```python
from build123d import *

# Parameters (mm, degrees)
ESBO_O1_W                  = 148
ESBO_O1_H                  = 130
RESSALTO_EXTRUS_O1_DEPTH   = 10
FURO_COM_FOLGA_DE_M3X0_5_D = 3.4
ESBO_O5_R                  = 5
CORTE_EXTRUS_O1_DEPTH      = 4.5
CORTE_EXTRUS_O2_REACH      = 205.463
ESBO_O6_R                  = 4


with BuildPart() as part:
    # Esboço1 → Ressalto-extrusão1 (new body)
    with BuildSketch(Plane.XY):
        with Locations((-0.0034, 124.2634)):
            Rectangle(ESBO_O1_W, ESBO_O1_H)
    extrude(amount=RESSALTO_EXTRUS_O1_DEPTH)

    # Furo com folga de M3X0.5 (through all)
    with Locations(Plane.XY.offset(10)):
        with Locations((38.5, 67), (-38.5068, 67), (65.5, 124), (-65.5068, 124), (-38.5068, 181), (38.5, 181)):
            Hole(FURO_COM_FOLGA_DE_M3X0_5_D / 2)

    # Esboço5 → Corte-extrusão1 (cut)
    with BuildSketch(Plane.XY.offset(10)):
        with Locations((-18.7634, 111.5234)):
            Circle(ESBO_O5_R)
        with Locations((18.8366, 137.5034)):
            Circle(ESBO_O5_R)
    extrude(amount=-CORTE_EXTRUS_O1_DEPTH, mode=Mode.SUBTRACT)

    # Esboço6 → Corte-extrusão2 (cut, up to next)
    with BuildSketch(Plane.XY.offset(10), mode=Mode.PRIVATE) as corte_extrus_o2_sk1:
        with Locations((-18.7634, 111.5234)):
            Circle(ESBO_O6_R)
    corte_extrus_o2_tool1 = extrude(corte_extrus_o2_sk1.sketch, amount=-CORTE_EXTRUS_O2_REACH, mode=Mode.PRIVATE) & part.part
    # Esboço6 → Corte-extrusão2 (cut, up to next)
    with BuildSketch(Plane.XY.offset(10), mode=Mode.PRIVATE) as corte_extrus_o2_sk2:
        with Locations((18.8366, 137.5034)):
            Circle(ESBO_O6_R)
    corte_extrus_o2_tool2 = extrude(corte_extrus_o2_sk2.sketch, amount=-CORTE_EXTRUS_O2_REACH, mode=Mode.PRIVATE) & part.part
    add(corte_extrus_o2_tool1.solids().sort_by_distance((-18.7634, 111.5234, 10))[0], mode=Mode.SUBTRACT)
    add(corte_extrus_o2_tool2.solids().sort_by_distance((18.8366, 137.5034, 10))[0], mode=Mode.SUBTRACT)


solid = part.part
```
Check sheet for the modelled part. Datum: model origin and axes. Units: mm. A direction names the side the tool comes from. Round coordinates to 2 decimals unless told otherwise and drop trailing zeros. Loops run counter-clockwise (first coordinate to the right, second up) from the corner with the lowest first, then second, coordinate; pieces in that order, holes last. Notation, with made-up numbers: (39.5, 28.25) -> (74.5, 28.25) arc R16 ccw to (74.5, 36.25) -> close; hole circle Ø4 at (18, -8.75). An arc over 180 degrees is marked (long way). Write item = value, one per line. Start each with the question number.
1) Release check for a two-part mould opening along Y. For faces 3 (the cylindrical face through (-19.28, 115.49, 2.79)), 4 (the flat face through (73.997, 123, 5)), 5 (the flat face through (-1, 189.263, 5)), 6 (the cylindrical face through (-63.81, 124.07, 4.93)) record: released by +Y, released by -Y, zero draft, split by the parting line, or undercut.
2) Sectioned sample at B-B, the plane y = 124. Record the cut outline in (x, z).
3) Sectioned sample at A-A, the plane x = 38.5. Record the cut outline in (y, z), plus the area to 3 significant figures.
4) Thickness scan on probe 1 along X at (y, z) = (124, 4.75); probe 2 along X at (y, z) = (181, 5); probe 3 along Y at (x, z) = (38.5, 5). Record the ranges inside material, lowest first.
5) Set-up check for faces 1 (the cylindrical face through (39.85, 65.97, 4.93)), 2 (the cylindrical face through (-16.08, 115.74, 7.78)): record each of +Z, -Z, +X, -X, +Y, -Y from which the full face is reachable in a straight line by a thin tool's end or side.
6) Sectioned sample at C-C, the plane x = 65.5. Record the cut outline in (y, z), plus the area to 3 significant figures.
Results are:
q1.face_3 = undercut
q1.face_4 = zero draft
q1.face_5 = released by +Y
q1.face_6 = undercut
q2.outline = (-74, 0) -> (-67.21, 0) -> (-67.21, 10) -> (-74, 10) -> close; (-63.81, 0) -> (63.8, 0) -> (63.8, 10) -> (-63.81, 10) -> close; (67.2, 0) -> (74, 0) -> (74, 10) -> (67.2, 10) -> close
q3.outline = (59.26, 0) -> (65.3, 0) -> (65.3, 10) -> (59.26, 10) -> close; (68.7, 0) -> (179.3, 0) -> (179.3, 10) -> (68.7, 10) -> close; (182.7, 0) -> (189.26, 0) -> (189.26, 10) -> (182.7, 10) -> close
q3.area = 1,230 mm^2
q4.probe_1 = -74 to -67.21, -63.81 to 63.8, 67.2 to 74
q4.probe_2 = -74 to -40.21, -36.81 to 36.8, 40.2 to 74
q4.probe_3 = 59.26 to 65.3, 68.7 to 179.3, 182.7 to 189.26
q5.face_1 = +Z, -Z
q5.face_2 = +Z
q6.outline = (59.26, 0) -> (122.3, 0) -> (122.3, 10) -> (59.26, 10) -> close; (125.7, 0) -> (189.26, 0) -> (189.26, 10) -> (125.7, 10) -> close
q6.area = 1,270 mm^2
